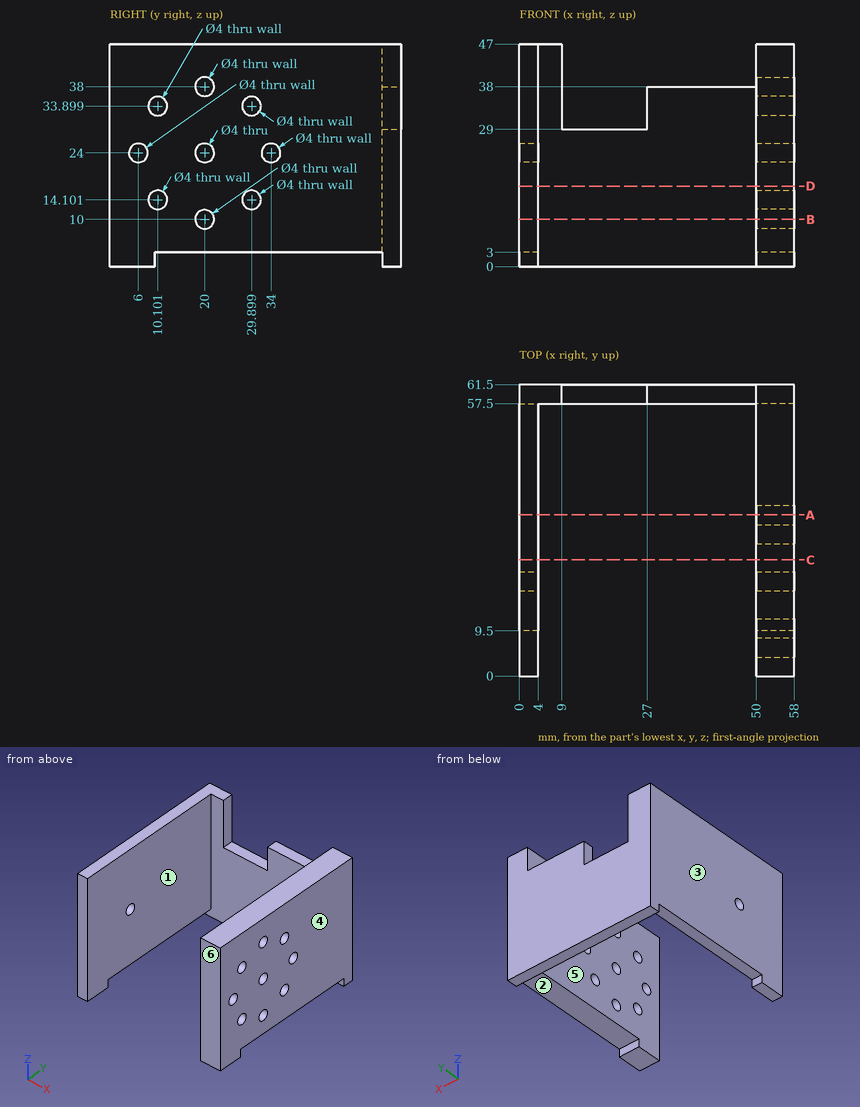
Geometry check sheet. Reference: drawing and pictorial views, mm from the part's lowest x, y, z. A direction names the side the tool comes from. Give positions to 0.01 mm unless a question says otherwise; leave off trailing zeros. Write each loop counter-clockwise with the first axis right and the second up, starting at its lowest first coordinate (ties: lowest second). Pieces come first, ordered by that corner, then holes. Notation, with made-up numbers: M 55,65.5 L 59,65.5 A22 cw 59,82.5 Z; hole C 37,85.5 d11. An arc over 180 degrees is marked long. Put each result on its own line as item: value. Start each with the question number.
1. Set-up check for the marked faces 1, 2 and 3: record each of +Z, -Z, +X, -X, +Y, -Y from which the full face is reachable in a straight line by a thin tool's end or side.
2. Section check C-C (y = 24.5). Record the cut outline in (x, z), and give its area (3 significant figures).
3. Draft check along X on the marked faces 4, 5 and 6. Enter one of: +X half, -X half, draft (parallel to the pull), parting line (faces both ways), or undercut.
4. Section check B-B (z = 10). Record the cut outline in (x, y).
5. Scan lines: line 1 along Y through (x, z) = (52.5, 10); line 2 along X through (y, z) = (9.5, 39); line 3 along Y through (x, z) = (52, 24). Record each from-to range of solid material in increasing order. Write a range as [from, to].
6. Go/stop test with flat-tipped pins: pin 1 Ø4.5 at (y, z) = (10.1, 14.1) entering from -X; pin 2 Ø2 at (x, y) = (15, 60) entering from +Z; pin 3 Ø6 at (x, z) = (12.5, 7) entering from -Y; pin 4 Ø6.5 at (x, y) = (54, 23) entering from -Z. Record where each tip stops, or that it passes through.
7. Section check D-D (z = 17). Record the cut outline in (x, y).
8. Section check A-A (y = 34). Record the cut outline in (x, z), and give its area (3 significant figures).
Answer list:
1. face 1: +Z, -Z, -Y
1. face 2: -Z, +X, -X
1. face 3: +Z, -Z, -X, +Y, -Y
2. outline: M 0,3 L 4,3 L 4,47 L 0,47 Z; M 50,3 L 58,3 L 58,47 L 50,47 Z
2. area: 528 mm2
3. face 4: +X half
3. face 5: undercut
3. face 6: draft
4. outline: M 0,0 L 4,0 L 4,57.5 L 50,57.5 L 50,22 L 58,22 L 58,61.5 L 0,61.5 Z; M 50,0 L 58,0 L 58,18 L 50,18 Z
5. line 1: [0, 18], [22, 61.5]
5. line 2: [0, 4], [50, 58]
5. line 3: [0, 4], [8, 18], [22, 32], [36, 61.5]
6. pin 1: x = 0
6. pin 2: z = 29
6. pin 3: y = 57.5
6. pin 4: z = 3
7. outline: M 0,0 L 4,0 L 4,57.5 L 50,57.5 L 50,0 L 58,0 L 58,61.5 L 0,61.5 Z
8. outline: M 0,3 L 4,3 L 4,47 L 0,47 Z; M 50,3 L 58,3 L 58,22 L 50,22 Z; M 50,26 L 58,26 L 58,47 L 50,47 Z
8. area: 496 mm2
